The listing builds one solid part. Answer for the finished solid, in the listing's coordinates (mm). A direction names the side the tool comes from. Round coordinates to 2 decimals unless told otherwise and drop trailing zeros. Write each loop counter-clockwise with the first axis right and the second up, starting at its lowest first coordinate (ties: lowest second). Pieces come first, ordered by that corner, then holes. Notation, with made-up numbers: M 10.5,27 L 27.5,27 A22 cw 27.5,39 Z; hole C 50,67 d10. An arc over 180 degrees is marked long. One line per item, written item: value. Start each with the question number.
(1) For a pull along X with two mould halves and no side action, classify faces 1 (the cylindrical face through (-0.06, 2.16, 7.51)), 2 (the flat face through (-1.05, -3, 8)), 3 (the flat face through (1, -3, 17.272)), 4 (the flat face through (1, -3, 15.24)) as released by +X, released by -X, zero draft, split by the parting line, or undercut.
(2) Given P1, Ø1, axis at y = -4, z = 9, coming from the -X side, flat-ended and moving along its own axis, determine where the tip first touches the part or whether it passes through.
(3) For faces 5 (the cylindrical face through (4.536, -2.766, 7.513)), 6 (the cylindrical face through (-3.14, 0.56, 16.24)), determine the directions among +Z, -Z, +X, -X, +Y, -Y from which every point of the face is accessible in a straight line to the end or side of a thin tool.
(4) Section C-C (z = 13.75) is taken. Determine the outline of the cut face in (x, y), plus the area to 3 significant figures.
(5) Consider probe 1 along X at (y, z) = (-3, 9); probe 2 along Z at (x, y) = (2, -3); probe 3 along Y at (x, z) = (3, 9.25). Determine where each line is inside the solid, lowest interval first.
```python
from build123d import *

# Parameters (mm, degrees)
F0_R     = 5.08
F1_DEPTH = 15.24
F3_R     = 5.08
F4_DEPTH = 2.032


with BuildPart() as f1:
    # F0 (on Top) → F1 (new body)
    with BuildSketch(Plane.XY):
        with Locations((0.600746, -2.876205)):
            Circle(F0_R)
        with BuildLine():
            Line((-1.050254, -6.450302), (-1.050254, -2.876205))
            Line((-1.050254, -2.876205), (-1.050254, 0.697892))
            ThreePointArc((-1.050254, 0.697892), (4.537746, -2.876205), (-1.050254, -6.450302))
        make_face(mode=Mode.SUBTRACT)
    extrude(amount=F1_DEPTH)

    # F3 (on offset) → F4 (join)
    with BuildSketch(Plane.XY.offset(15.24)):
        with Locations((0.600743, -2.876237)):
            Circle(F3_R)
    extrude(amount=F4_DEPTH)


solid = f1.part
```
Recorded:
1. face 1: split by the parting line
1. face 2: undercut
1. face 3: zero draft
1. face 4: undercut
2. P1: stops at x = -4.44
3. face 5: -Z
3. face 6: +Z, -Z
4. outline: C 0.6,-2.88 d10.16; hole M -1.05,-6.45 A3.94 ccw long -1.05,0.7 Z
4. area: 44.1 mm2
5. probe 1: x = -4.48 to -1.05, 4.54 to 5.68
5. probe 2: z = 15.24 to 17.27
5. probe 3: y = -7.35 to -6, 0.25 to 1.6
